The listing builds one solid part. Answer for the finished solid, in the listing's coordinates (mm). Face numbers are marked on the shaded views. Give positions to 0.01 mm unless a question says otherwise; leave off trailing zeros. Order: outer loops, then holes, each group sorted by start corner. A loop starts at its lowest first (then second) coordinate and runs counter-clockwise, first axis right, second up. Notation, with made-up numbers: (21, 70) - (39, 70) arc R25 cw to (39, 104) - close; hole circle Ø10 at (69, 86.25). An arc over 180 degrees is marked (long way). Use a Markdown table: item, result. Add a question column.
1) Straight lines are drawn through the part: line 1 (X direction, y = 11.5, z = -8.5); line 2 (Z direction, x = -13.5, y = -6.7); line 3 (Z direction, x = 13, y = -1). For each, find the intervals that lie inside material, in ascending order.
2) The mould has two halves that part along Z. Classify the marked faces 1, 2 and 3: released by +Z, released by -Z, zero draft, split by the parting line, or undercut.
3) Find section D-D, the plane z = -50. Determine the outline of the cut face in (x, y).
4) Find section A-A, the plane z = 62. Determine the outline of the cut face in (x, y), plus the area to 3 significant figures.
5) Find section C-C, the plane y = 35. Determine the outline of the cut face in (x, z), plus the area to 3 significant figures.
6) Flat-ended cylindrical pins translate along their axes: pin 1 (1 mm diameter, centred on x = -10.5, z = 31, fed in from +Y); pin 2 (5 mm diameter, centred on x = -14.5, z = -48.5, fed in from +Y); pin 3 (3 mm diameter, centred on x = 16, z = -70.5, fed in from +Y); pin 4 (6 mm diameter, centred on x = -22.5, y = 16, fed in from -Z). Find the tip coordinate at first contact, or state that the pin passes through.
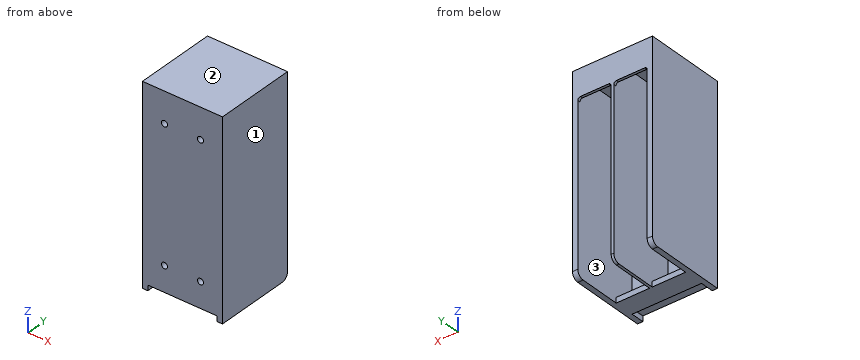
Autodesk Fusion 360 part; units mm, degrees
sketch "Sketch1" plane through (0, 0, 0) normal (0, 1, 0) x (1, 0, 0)
  line L0 (-30, 73) -> (30, 73)
  line L1 (30, 73) -> (30, -73)
  line L2 (30, -73) -> (-30, -73)
  line L3 (-30, -73) -> (-30, 73)
  line L4 (-26, 69) -> (-1, 69)
  line L5 (-1, 69) -> (-1, -69)
  line L6 (-1, -69) -> (-26, -69)
  line L7 (-26, -69) -> (-26, 69)
  line L8 (-26, 69) -> (26, 69)
  line L9 (26, 69) -> (26, -69)
  line L10 (26, -69) -> (-26, -69)
  line L11 (-26, -69) -> (-26, 69)
  line L12 (30, -73) -> (-30, 73) construction
  line L13 (26, 69) -> (1, 69)
  line L14 (1, 69) -> (1, -69)
  line L15 (26, -64) -> (26, 69)
  line L16 (-26, 69) -> (-26, 73)
  line L17 (26, 69) -> (26, 73)
  line L18 (-1, 69) -> (-1, 73)
  line L19 (1, 69) -> (1, 73)
  dimension "d1" = 60
  dimension "d2" = 146
  dimension "d3" = 25
  dimension "d4" = 138
  dimension "d5" = 4
  dimension "d6" = 25
  dimension "d7" = 133
extrude "Extrude1" add sketch "Sketch1" along normal blind 49 contours L0 L1 L2 L3 L6 L7 L9 L10 L11 L15 L16 L17 | L0 L8 L18 L19 | L5 L8 L10 L14
extrude "Extrude2" add sketch "Sketch1" against normal blind 10 contours L0 L1 L2 L3 L6 L7 L9 L10 L11 L15 L16 L17 | L4 L5 L6 L7 L8 L10 L11 | L5 L8 L10 L14 | L8 L9 L10 L13 L14 L15
extrude "Extrude3" add sketch "Sketch1" along normal blind 15 contours L0 L4 L8 L16 L18 | L0 L8 L13 L17 L19
sketch "Sketch2" plane through (0, 49, 0) normal (0, 1, 0) x (-1, 0, 0)
  line L0 (-1, 69) -> (-1, -73)
  line L1 (-1, -73) -> (1, -73)
  line L2 (1, -73) -> (1, 69)
  line L3 (1, 69) -> (26, 69)
  line L4 (26, 69) -> (26, -73)
  line L5 (26, -73) -> (30, -73)
  line L6 (30, -73) -> (30, 73)
  line L7 (30, 73) -> (-30, 73)
  line L8 (-30, 73) -> (-30, -73)
  line L9 (-30, -73) -> (-26, -73)
  line L10 (-26, -73) -> (-26, 69)
  line L11 (-26, 69) -> (-1, 69)
  line L12 (30, 73) -> (-30, 73)
  line L13 (-30, 73) -> (-30, 53)
  line L14 (-30, 53) -> (30, 53)
  line L15 (30, 53) -> (30, 73)
  dimension "d14" = 20
extrude "Extrude4" add sketch "Sketch2" along normal blind 2 contours L0 L2 L3 L4 L6 L7 L8 L10 L11 L12 L13 L14 L15 | L0 L10 L11 L14 | L2 L3 L4 L14
extrude "Extrude5" add 3 faces at (28.6667, 49, 11) (0.3333, 49, -31) (-28.6667, 49, 11) along direction (0, 1, 0) blind 2
fillet "Fillet1" radius 5 3 edges at (28, 51, -73) (0, 51, -73) (-28, 51, -73)
fillet "Fillet2" radius 2 4 edges at (1, 50, 53) (-26, 50, 53) (-1, 50, 53) (26, 50, 53)
sketch "Sketch3" plane through (0, 0, 0) normal (0, 1, 0) x (-1, 0, 0)
  line L0 (1, -69) -> (26, -69)
  line L1 (26, -69) -> (26, 69)
  line L2 (26, 69) -> (1, 69)
  line L3 (1, 69) -> (1, -69)
  circle A0 centre (13.5, -50) radius 2.25
  circle A1 centre (13.5, 50) radius 2.25
  line L4 (13.5, -50) -> (13.5, 50)
  line L5 (26, 0) -> (1, 0)
  dimension "d24" = 4.5
  dimension "d26" = 4.5
  dimension "d43" = 100
extrude "Extrude6" cut sketch "Sketch3" against normal blind 10 contours A0 | A1
sketch "Sketch4" plane through (0, 0, 0) normal (0, 1, 0) x (-1, 0, 0)
  circle A0 centre (13.5, -50) radius 2.25
  circle A1 centre (13.5, 50) radius 2.25
  line L0 (1, -69) -> (26, -69)
  line L1 (26, -69) -> (26, 69)
  line L2 (26, 69) -> (1, 69)
  line L3 (1, 69) -> (1, -69)
  circle A2 centre (13.5, -50) radius 5
  circle A3 centre (13.5, 50) radius 5
  dimension "d29" = 10
  dimension "d30" = 10
extrude "Extrude7" cut sketch "Sketch4" against normal blind 5 contours A2 | A3
sketch "Sketch5" plane through (0, 0, 0) normal (0, 1, 0) x (-1, 0, 0)
  line L0 (-26, -69) -> (-1, -69)
  line L1 (-1, -69) -> (-1, 69)
  line L2 (-1, 69) -> (-26, 69)
  line L3 (-26, 69) -> (-26, -69)
  circle A0 centre (-13.5, -50) radius 2.25
  circle A1 centre (-13.5, 50) radius 2.25
  circle A2 centre (-13.5, -50) radius 5
  circle A3 centre (-13.5, 50) radius 5
  line L4 (-13.5, 50) -> (-13.5, -50)
  line L5 (-1, 0) -> (-26, 0)
  dimension "d35" = 4.5
  dimension "d36" = 4.5
  dimension "d37" = 10
  dimension "d38" = 10
  dimension "d44" = 100
extrude "Extrude8" cut sketch "Sketch5" against normal blind 10 contours A0 | A1
extrude "Extrude9" cut sketch "Sketch5" against normal blind 5 contours A2 | A3
equation "d1 = ( 25 * 2 ) * 1 mm + 10 mm"
equation "d2 = 138 mm + 8 mm"
The answers:
| question | item | result |
|---|---|---|
| 1 | line 1 | -30 to -26, -1 to 1, 26 to 30 |
| 1 | line 2 | -69 to -52.25, -47.75 to 47.75, 52.25 to 73 |
| 1 | line 3 | -69 to -54.97, -45.03 to 45.03, 54.97 to 73 |
| 2 | face 1 | zero draft |
| 2 | face 2 | released by +Z |
| 2 | face 3 | undercut |
| 3 | outline | (-30, -10) - (-15.75, -10) - (-15.75, -5) - (-18.5, -5) - (-18.5, 0) - (-26, 0) - (-26, 51) - (-30, 51) - close; (-11.25, -10) - (11.25, -10) - (11.25, -5) - (8.5, -5) - (8.5, 0) - (1, 0) - (1, 51) - (-1, 51) - (-1, 0) - (-8.5, 0) - (-8.5, -5) - (-11.25, -5) - close; (15.75, -10) - (30, -10) - (30, 51) - (26, 51) - (26, 0) - (18.5, 0) - (18.5, -5) - (15.75, -5) - close |
| 4 | outline | (-30, -10) - (30, -10) - (30, 51) - (-30, 51) - close; hole (-26, 0) - (-1, 0) - (-1, 49) - (-26, 49) - close; hole (1, 0) - (26, 0) - (26, 49) - (1, 49) - close |
| 4 | area | 1,210 mm2 |
| 5 | outline | (-30, -73) - (-26, -73) - (-26, 69) - (-1, 69) - (-1, -73) - (1, -73) - (1, 69) - (26, 69) - (26, -73) - (30, -73) - (30, 73) - (-30, 73) - close |
| 5 | area | 1,660 mm2 |
| 6 | pin 1 | y = 0 |
| 6 | pin 2 | y = -5 |
| 6 | pin 3 | y = 15 |
| 6 | pin 4 | z = -73 |
